```python
from build123d import *

# Parameters (mm, degrees)
SKETCH_2_R      = 29
EXTRUDE_1_DEPTH = 66
SKETCH_2_3_R    = 36
EXTRUDE_2_DEPTH = 58
EXTRUDE_START   = 50
SKETCH_2_4_R    = 42
SKETCH_2_4_R_2  = 36
EXTRUDE_3_DEPTH = 5


with BuildPart() as part:
    # 草图2 → 凸台-拉伸1 (new body)
    with BuildSketch(Plane(origin=(0, 0, 0), x_dir=(1, 0, 0), z_dir=(0, 1, 0))):
        with Locations((-35.483898972, -6.127114057)):
            Circle(SKETCH_2_R)
    extrude(amount=EXTRUDE_1_DEPTH)

    # 草图2<3> → 凸台-拉伸2 (add)
    with BuildSketch(Plane(origin=(0, 0, 0), x_dir=(1, 0, 0), z_dir=(0, 1, 0))):
        with Locations((-35.483898972, -6.127114057)):
            Circle(SKETCH_2_3_R)
    extrude(amount=EXTRUDE_2_DEPTH)

    # 草图2<4> → 凸台-拉伸3 (add)
    with BuildSketch(Plane(origin=(0, 0, 0), x_dir=(1, 0, 0), z_dir=(0, 1, 0)).offset(EXTRUDE_START)):
        with Locations((-35.483898972, -6.127114057)):
            Circle(SKETCH_2_4_R)
        with Locations((-35.483898972, -6.127114057)):
            Circle(SKETCH_2_4_R_2, mode=Mode.SUBTRACT)
    extrude(amount=EXTRUDE_3_DEPTH)


solid = part.part
```
Input: part model. Units: mm. Frame: model coordinates. A direction names the side the tool comes from. Round coordinates to 2 decimals unless told otherwise and drop trailing zeros. Loops run counter-clockwise (first coordinate to the right, second up) from the corner with the lowest first, then second, coordinate; pieces in that order, holes last. Notation, with made-up numbers: (-20, 35.25) -> (10, 35.25) arc R25 ccw to (10, 72.25) -> close; hole circle Ø9 at (65.25, -33.5). An arc over 180 degrees is marked (long way). One line per item, written item: value.
(1) Set-up query: faces 1 (the face through (-4.6, 50, -12.7)), 2 (the face through (-71.45, 56.48, 4.54)), 3 (the face through (4.577, 52.465, -6.489)). Return all of +Z, -Z, +X, -X, +Y, -Y with unobstructed straight access to the full face (end or side cutting, diameter ignored); none if empty.
Geometry check:
face 1: -Y
face 2: +Y
face 3: +Y, -Y
(2) Section A-A (z = -2). Return the cut outline in (x, y), plus the area to 3 significant figures.
Geometry check:
outline: (-76.69, 50) -> (-70.55, 50) -> (-70.55, 0) -> (-0.41, 0) -> (-0.41, 50) -> (5.72, 50) -> (5.72, 55) -> (-0.41, 55) -> (-0.41, 58) -> (-7.65, 58) -> (-7.65, 66) -> (-63.32, 66) -> (-63.32, 58) -> (-70.55, 58) -> (-70.55, 55) -> (-76.69, 55) -> close
area: 4,570 mm2
(3) Section C-C (y = 34). Return the cut outline in (x, z).
Geometry check:
outline: circle Ø72 at (-35.48, 6.13)
(4) Section B-B (x = -29.5). Return the cut outline in (y, z), plus the area to 3 significant figures.
Geometry check:
outline: (0, -29.37) -> (50, -29.37) -> (50, -35.44) -> (55, -35.44) -> (55, -29.37) -> (58, -29.37) -> (58, -22.25) -> (66, -22.25) -> (66, 34.5) -> (58, 34.5) -> (58, 41.63) -> (55, 41.63) -> (55, 47.7) -> (50, 47.7) -> (50, 41.63) -> (0, 41.63) -> close
area: 4,630 mm2
(5) Material intervals for line 1 (Y direction, x = -64, z = 17); line 2 (Y direction, x = -49.5, z = -30.5); line 3 (X direction, y = 29.5, z = 3.5), sorted ascending. Write a range as [from, to].
Geometry check:
line 1: [0, 58]
line 2: [50, 55]
line 3: [-71.39, 0.42]
(6) Pin query (flat end, axial travel): pin 1 (2 mm diameter, centred on x = -10, y = 54.5, fed in from -Z); pin 2 (3 mm diameter, centred on x = -69, y = 23.5, fed in from +Z); pin 3 (2 mm diameter, centred on x = -3, y = 27, fed in from +Z); pin 4 (2 mm diameter, centred on x = -60.5, z = -9, fed in from +Y). Return the tip coordinate at first contact, or that it passes through.
Geometry check:
pin 1: z = -28
pin 2: z = 22.59
pin 3: z = 23.58
pin 4: y = 66
(7) Section D-D (x = -4). Return the cut outline in (y, z), plus the area to 3 significant figures.
Geometry check:
outline: (0, -11.33) -> (50, -11.33) -> (50, -21.67) -> (55, -21.67) -> (55, -11.33) -> (58, -11.33) -> (58, 23.58) -> (55, 23.58) -> (55, 33.93) -> (50, 33.93) -> (50, 23.58) -> (0, 23.58) -> close
area: 2,130 mm2
